Read the model definition and answer for the solid it produces. Units are mm, in the model's axes. A direction names the side the tool comes from. Give positions to 0.01 mm unless a question says otherwise; leave off trailing zeros. Loops run counter-clockwise (first coordinate to the right, second up) from the corner with the lowest first, then second, coordinate; pieces in that order, holes last.
(1) Which of the six approach directions +Z, -Z, +X, -X, +Y, -Y give full straight-line access (tool end or side, diameter ignored) to faces 1 (the face through (-4.88, 0.74, -1.08)), 2 (the face through (6.44, 3.23, -0.35))?
(2) Straight lines are drawn through the part: probe 1 along X at (y, z) = (3.15, 0); probe 2 along Y at (x, z) = (-5.5, 2.25); probe 3 along X at (y, z) = (3.3, -8). For each, find the intervals that lie inside material, in ascending order.
(3) Find section C-C, the plane x = -2.5. Write down the section's boundary in (y, z), then the cut area to 3 significant figures.
(4) Find section B-B, the plane z = 0. Write down the section's boundary in (x, y).
(5) Find section A-A, the plane x = 0. Write down the section's boundary in (y, z).
(6) Determine the mould class of faces 3 (the face through (-3.905, 7.395, -0.867)), 4 (the face through (-4.88, 9.93, -1.08)), 5 (the face through (-5, 5, 2)) for opening direction X: pulls with the +X half, pulls with the -X half, needs draft (parallel to the pull), parting line crosses it, or undercut.
(7) Find section D-D, the plane z = -3.5. Write down the section's boundary in (x, y), then the cut area to 3 significant figures.
(8) Each of these flat-tipped pins is pushed along its axis until it touches: P1, Ø8, axis at y = 5.5, z = 5.5, coming from the +X side; P2, Ø1, axis at x = 8.5, z = -1.5, coming from the -Y side; P3, Ø3.5, axis at x = -8, z = 0, coming from the +Y side; P4, Ø2.5, axis at x = 0, z = -8, coming from the +Y side. Where does it stop, or does it pass through?
```python
from build123d import *

# Parameters (mm, degrees)
SKETCH_1_R      = 5
SKETCH_1_R_2    = 4
EXTRUDE_1_DEPTH = 15
EXTRUDE_START   = 1.5
SKETCH_2_R      = 11
SKETCH_2_R_2    = 5
SKETCH_2_R_3    = 1.6
EXTRUDE_2_DEPTH = 3.5


with BuildPart() as part:
    # 草图1 → 凸台-拉伸1 (new body)
    with BuildSketch(Plane(origin=(0, 0, 0), x_dir=(1, 0, 0), z_dir=(0, 1, 0))):
        with Locations(Location((0, 0, 0), (0, 0, 270))):
            Circle(SKETCH_1_R)
        with Locations(Location((0, 0, 0), (0, 0, 270))):
            Circle(SKETCH_1_R_2, mode=Mode.SUBTRACT)
    extrude(amount=EXTRUDE_1_DEPTH)

    # 草图2 → 凸台-拉伸2 (add)
    with BuildSketch(Plane(origin=(0, 0, 0), x_dir=(1, 0, 0), z_dir=(0, 1, 0)).offset(EXTRUDE_START)):
        with Locations(Location((0, 0, 0), (0, 0, 270))):
            Circle(SKETCH_2_R)
        with Locations(Location((0, 0, 0), (0, 0, 270))):
            Circle(SKETCH_2_R_2, mode=Mode.SUBTRACT)
        with Locations(Location((0, 8, 0), (0, 0, 270))):
            Circle(SKETCH_2_R_3, mode=Mode.SUBTRACT)
        with Locations(Location((8, 0, 0), (0, 0, 270))):
            Circle(SKETCH_2_R_3, mode=Mode.SUBTRACT)
        with Locations(Location((0, -8, 0), (0, 0, 270))):
            Circle(SKETCH_2_R_3, mode=Mode.SUBTRACT)
        with Locations(Location((-8, 0, 0), (0, 0, 270))):
            Circle(SKETCH_2_R_3, mode=Mode.SUBTRACT)
    extrude(amount=EXTRUDE_2_DEPTH)


solid = part.part
```
Entries:
1. face 1: -Y
1. face 2: +Y, -Y
2. probe 1: x = -11 to -9.6, -6.4 to -4, 4 to 6.4, 9.6 to 11
2. probe 2: y = 1.5 to 5
2. probe 3: x = -7.55 to -1.6, 1.6 to 7.55
3. outline: (0, -4.33) - (1.5, -4.33) - (1.5, -10.71) - (5, -10.71) - (5, -4.33) - (15, -4.33) - (15, -3.12) - (0, -3.12) - close; (0, 3.12) - (15, 3.12) - (15, 4.33) - (5, 4.33) - (5, 10.71) - (1.5, 10.71) - (1.5, 4.33) - (0, 4.33) - close
3. area: 80.9 mm2
4. outline: (-11, 1.5) - (-9.6, 1.5) - (-9.6, 5) - (-11, 5) - close; (-6.4, 1.5) - (-5, 1.5) - (-5, 0) - (-4, 0) - (-4, 15) - (-5, 15) - (-5, 5) - (-6.4, 5) - close; (4, 0) - (5, 0) - (5, 1.5) - (6.4, 1.5) - (6.4, 5) - (5, 5) - (5, 15) - (4, 15) - close; (9.6, 1.5) - (11, 1.5) - (11, 5) - (9.6, 5) - close
5. outline: (0, -5) - (1.5, -5) - (1.5, -6.4) - (5, -6.4) - (5, -5) - (15, -5) - (15, -4) - (0, -4) - close; (0, 4) - (15, 4) - (15, 5) - (5, 5) - (5, 6.4) - (1.5, 6.4) - (1.5, 5) - (0, 5) - close; (1.5, -11) - (5, -11) - (5, -9.6) - (1.5, -9.6) - close; (1.5, 9.6) - (5, 9.6) - (5, 11) - (1.5, 11) - close
6. face 3: undercut
6. face 4: parting line crosses it
6. face 5: needs draft
7. outline: (-10.43, 1.5) - (-3.57, 1.5) - (-3.57, 0) - (-1.94, 0) - (-1.94, 15) - (-3.57, 15) - (-3.57, 5) - (-10.43, 5) - close; (1.94, 0) - (3.57, 0) - (3.57, 1.5) - (10.43, 1.5) - (10.43, 5) - (3.57, 5) - (3.57, 15) - (1.94, 15) - close
7. area: 97.0 mm2
8. P1: stops at x = 10.89
8. P2: stops at y = 1.5
8. P3: stops at y = 5
8. P4: passes through
